The listing builds one solid part. Answer for the finished solid, in the listing's coordinates (mm). A direction names the side the tool comes from. Round coordinates to 2 decimals unless told otherwise and drop trailing zeros. Write each loop counter-clockwise with the first axis right and the second up, starting at its lowest first coordinate (ties: lowest second). Pieces come first, ordered by that corner, then holes.
Item 1: Each of these flat-tipped pins is pushed along its axis until it touches: pin 1 (0.9 mm diameter, centred on x = -67, y = 2, fed in from +Z); pin 2 (1.5 mm diameter, centred on y = 1, z = 27.5, fed in from +X); pin 3 (2.5 mm diameter, centred on x = 49, z = 30, fed in from +Y). Where does it stop, or does it pass through?
Item 2: Find the intervals of material crossed by probe 1 along X at (y, z) = (1.55, 30); probe 2 along X at (y, z) = (2.25, -32); probe 3 along Z at (x, y) = (-80, 1.5), in increasing order.
Item 3: For a pull along X with two mould halves and no side action, classify faces 1 (the face through (30.615, 1.521, 30.784)), 2 (the face through (-73, 1, 14.25)), 3 (the face through (52, 1, 38)) as +X half, -X half, draft (parallel to the pull), parting line (faces both ways), or undercut.
Item 4: A tool of negligible diameter and unlimited length cuts with its end or side. For faces 4 (the face through (30.5, 1, 0)), 5 (the face through (-55, 1, 24)), 6 (the face through (-55, 1, -25)), from which of +Z, -Z, +X, -X, +Y, -Y can it reach the whole face along a straight path? Write none if from no direction.
Item 5: Find section D-D on y = 0.7. Give the number of separate pieces and of enclosed holes in the cut face, then the cut area to 3 significant figures.
Item 6: Find section B-B on z = 20. Give the vertices of the cut face in (x, y), then the cut area to 3 significant figures.
Item 7: Find section C-C on x = 19.5. Give the vertices of the cut face in (y, z).
Item 8: Find section A-A on x = 80. Give the vertices of the cut face in (y, z).
```python
from build123d import *

# Parameters (mm, degrees)
SKETCH1_W           = 19
SKETCH1_H           = 46
SKETCH1_W_2         = 16
SKETCH1_H_2         = 36
SKETCH1_R           = 1.7
BOSS_EXTRUDE1_DEPTH = 3
SKETCH4_R           = 1.65
CUT_EXTRUDE2_DEPTH  = 15
SKETCH5_R           = 1.65
CUT_EXTRUDE3_DEPTH  = 10
CHAMFER1_SIZE       = 5


with BuildPart() as part:
    # Sketch1 → Boss-Extrude1 (new body)
    with BuildSketch(Plane(origin=(0, 0, 0), x_dir=(1, 0, 0), z_dir=(0, 1, 0))):
        Polygon((55, 40), (-55, 40), (-55, 14.25), (-90, 14.25), (-90, -14.25), (-55, -14.25), (-55, -40), (55, -40), (55, -14.25), (90, -14.25), (90, 14.25), (55, 14.25), align=None)
        Rectangle(SKETCH1_W, SKETCH1_H, mode=Mode.SUBTRACT)
        with Locations((22.5, 0)):
            Rectangle(SKETCH1_W_2, SKETCH1_H_2, mode=Mode.SUBTRACT)
        with Locations(Location((-66, 7, 0), (0, 0, 270))):
            Circle(SKETCH1_R, mode=Mode.SUBTRACT)
        with Locations(Location((-66, -7, 0), (0, 0, 270))):
            Circle(SKETCH1_R, mode=Mode.SUBTRACT)
        with Locations(Location((-80, -7, 0), (0, 0, 270))):
            Circle(SKETCH1_R, mode=Mode.SUBTRACT)
        with Locations(Location((-80, 7, 0), (0, 0, 270))):
            Circle(SKETCH1_R, mode=Mode.SUBTRACT)
        with Locations(Location((66, 7, 0), (0, 0, 270))):
            Circle(SKETCH1_R, mode=Mode.SUBTRACT)
        with Locations(Location((80, 7, 0), (0, 0, 270))):
            Circle(SKETCH1_R, mode=Mode.SUBTRACT)
        with Locations(Location((80, -7, 0), (0, 0, 270))):
            Circle(SKETCH1_R, mode=Mode.SUBTRACT)
        with Locations(Location((66, -7, 0), (0, 0, 270))):
            Circle(SKETCH1_R, mode=Mode.SUBTRACT)
    extrude(amount=BOSS_EXTRUDE1_DEPTH)

    # Sketch4 → Cut-Extrude2 (cut)
    with BuildSketch(Plane(origin=(0, 3, 0), x_dir=(1, 0, 0), z_dir=(0, 1, 0))):
        with Locations(Location((29.5, 32, 0), (0, 0, 270))):
            Circle(SKETCH4_R)
        with Locations(Location((19.5, 32, 0), (0, 0, 270))):
            Circle(SKETCH4_R)
        with Locations(Location((19.5, -32, 0), (0, 0, 270))):
            Circle(SKETCH4_R)
        with Locations(Location((29.5, -32, 0), (0, 0, 270))):
            Circle(SKETCH4_R)
        with Locations(Location((-19.5, 32, 0), (0, 0, 270))):
            Circle(SKETCH4_R)
        with Locations(Location((-29.5, 32, 0), (0, 0, 270))):
            Circle(SKETCH4_R)
        with Locations(Location((-29.5, -32, 0), (0, 0, 270))):
            Circle(SKETCH4_R)
        with Locations(Location((-19.5, -32, 0), (0, 0, 270))):
            Circle(SKETCH4_R)
    extrude(amount=-CUT_EXTRUDE2_DEPTH, mode=Mode.SUBTRACT)

    # Sketch5 → Cut-Extrude3 (cut)
    with BuildSketch(Plane(origin=(0, 3, 0), x_dir=(1, 0, 0), z_dir=(0, 1, 0))):
        with Locations(Location((-49, 30, 0), (0, 0, 270))):
            Circle(SKETCH5_R)
        with Locations(Location((-49, -20, 0), (0, 0, 270))):
            Circle(SKETCH5_R)
        with Locations(Location((-49, -30, 0), (0, 0, 270))):
            Circle(SKETCH5_R)
        with Locations(Location((-49, 20, 0), (0, 0, 270))):
            Circle(SKETCH5_R)
        with Locations(Location((49, 20, 0), (0, 0, 270))):
            Circle(SKETCH5_R)
        with Locations(Location((49, -30, 0), (0, 0, 270))):
            Circle(SKETCH5_R)
        with Locations(Location((49, -20, 0), (0, 0, 270))):
            Circle(SKETCH5_R)
        with Locations(Location((49, 30, 0), (0, 0, 270))):
            Circle(SKETCH5_R)
    extrude(amount=-CUT_EXTRUDE3_DEPTH, mode=Mode.SUBTRACT)

    # Chamfer1
    chamfer1_edges = [part.edges().sort_by_distance(p)[0] for p in [
        (55, 1.5, -40),
        (55, 1.5, 40),
        (-55, 1.5, 40),
        (-55, 1.5, -40),
    ]]
    chamfer(chamfer1_edges, length=CHAMFER1_SIZE)


solid = part.part
```
Check values:
1. pin 1: stops at z = 14.25
1. pin 2: stops at x = 55
1. pin 3: passes through
2. probe 1: x = -55 to -50.65, -47.35 to 47.35, 50.65 to 55
2. probe 2: x = -55 to -31.15, -27.85 to -21.15, -17.85 to 17.85, 21.15 to 27.85, 31.15 to 55
2. probe 3: z = -14.25 to -8.7, -5.3 to 5.3, 8.7 to 14.25
3. face 1: undercut
3. face 2: draft
3. face 3: +X half
4. face 4: +Y, -Y
4. face 5: +Z, -X, +Y, -Y
4. face 6: -Z, -X, +Y, -Y
5. separate pieces: 1
5. enclosed holes: 26
5. area: 9,090 mm2
6. outline: (-55, 0) - (-50.65, 0) - (-50.65, 3) - (-55, 3) - close; (-47.35, 0) - (-9.5, 0) - (-9.5, 3) - (-47.35, 3) - close; (9.5, 0) - (47.35, 0) - (47.35, 3) - (9.5, 3) - close; (50.65, 0) - (55, 0) - (55, 3) - (50.65, 3) - close
6. area: 253 mm2
7. outline: (0, -40) - (3, -40) - (3, -33.65) - (0, -33.65) - close; (0, -30.35) - (3, -30.35) - (3, -18) - (0, -18) - close; (0, 18) - (3, 18) - (3, 30.35) - (0, 30.35) - close; (0, 33.65) - (3, 33.65) - (3, 40) - (0, 40) - close
8. outline: (0, -14.25) - (3, -14.25) - (3, -8.7) - (0, -8.7) - close; (0, -5.3) - (3, -5.3) - (3, 5.3) - (0, 5.3) - close; (0, 8.7) - (3, 8.7) - (3, 14.25) - (0, 14.25) - close
